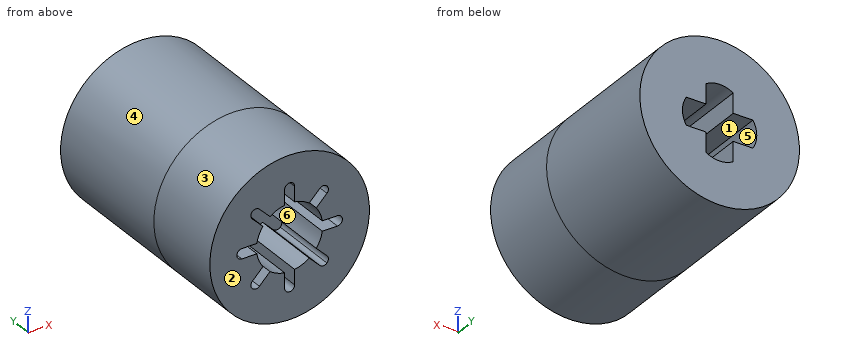
Autodesk Inventor part; units mm, degrees
ref_plane "YZ Plane" through (0, 0, 0) normal (1, 0, 0) x (0, 1, 0)
ref_plane "XZ Plane" through (0, 0, 0) normal (0, 1, 0) x (-1, 0, 0)
ref_plane "XY Plane" through (0, 0, 0) normal (0, 0, 1) x (1, 0, 0)
sketch "Sketch1" plane through (0, 0, 0) normal (0, 1, 0) x (-1, 0, 0)
  arc A0 (0, 3.7886) -> (-0.36, 3.4286) centre (0, 3.4286) ccw
  arc A1 (0.36, 3.4286) -> (0, 3.7886) centre (0, 3.4286) ccw
  line L0 (0, 3.7886) -> (0, 3.7886)
  line L1 (-2.6789, 2.1698) -> (-1.9152, 1.4061)
  arc A2 (-2.1698, 2.6789) -> (-2.6789, 2.6789) centre (-2.4244, 2.4244) ccw
  line L2 (-2.6789, 2.6789) -> (-2.6789, 2.6789)
  arc A3 (-2.6789, 2.6789) -> (-2.6789, 2.1698) centre (-2.4244, 2.4244) ccw
  line L3 (-3.4286, 0.36) -> (-2.3486, 0.36)
  arc A4 (-2.3486, 0.36) -> (-2.3486, -0.36) centre (0, 0) ccw
  line L4 (-3.4286, -0.36) -> (-2.3486, -0.36)
  arc A5 (-3.4286, 0.36) -> (-3.7886, 0) centre (-3.4286, 0) ccw
  line L5 (-3.7886, 0) -> (-3.7886, 0)
  arc A6 (-3.7886, 0) -> (-3.4286, -0.36) centre (-3.4286, 0) ccw
  line L6 (-2.6789, -2.1698) -> (-1.9152, -1.4061)
  arc A7 (-2.6789, -2.1698) -> (-2.6789, -2.6789) centre (-2.4244, -2.4244) ccw
  line L7 (-2.6789, -2.6789) -> (-2.6789, -2.6789)
  arc A8 (-2.6789, -2.6789) -> (-2.1698, -2.6789) centre (-2.4244, -2.4244) ccw
  line L8 (-2.1698, -2.6789) -> (-1.4061, -1.9152)
  arc A9 (-1.9152, -1.4061) -> (-1.4061, -1.9152) centre (0, 0) ccw
  line L9 (-0.36, -3.4286) -> (-0.36, -2.3486)
  arc A10 (-0.36, -2.3486) -> (0.36, -2.3486) centre (0, 0) ccw
  arc A11 (-0.36, -3.4286) -> (0, -3.7886) centre (0, -3.4286) ccw
  line L10 (0, -3.7886) -> (0, -3.7886)
  arc A12 (0, -3.7886) -> (0.36, -3.4286) centre (0, -3.4286) ccw
  line L11 (0.36, -3.4286) -> (0.36, -2.3486)
  line L12 (2.1698, -2.6789) -> (1.4061, -1.9152)
  arc A13 (1.4061, -1.9152) -> (1.9152, -1.4061) centre (0, 0) ccw
  arc A14 (2.1698, -2.6789) -> (2.6789, -2.6789) centre (2.4244, -2.4244) ccw
  line L13 (2.6789, -2.6789) -> (2.6789, -2.6789)
  arc A15 (2.6789, -2.6789) -> (2.6789, -2.1698) centre (2.4244, -2.4244) ccw
  line L14 (2.6789, -2.1698) -> (1.9152, -1.4061)
  line L15 (3.4286, -0.36) -> (2.3486, -0.36)
  arc A16 (2.3486, -0.36) -> (2.3486, 0.36) centre (0, 0) ccw
  line L16 (3.4286, 0.36) -> (2.3486, 0.36)
  arc A17 (3.4286, -0.36) -> (3.7886, 0) centre (3.4286, 0) ccw
  line L17 (3.7886, 0) -> (3.7886, 0)
  arc A18 (3.7886, 0) -> (3.4286, 0.36) centre (3.4286, 0) ccw
  line L18 (2.6789, 2.1698) -> (1.9152, 1.4061)
  arc A19 (1.9152, 1.4061) -> (1.4061, 1.9152) centre (0, 0) ccw
  arc A20 (2.6789, 2.1698) -> (2.6789, 2.6789) centre (2.4244, 2.4244) ccw
  line L19 (2.6789, 2.6789) -> (2.6789, 2.6789)
  arc A21 (2.6789, 2.6789) -> (2.1698, 2.6789) centre (2.4244, 2.4244) ccw
  line L20 (2.1698, 2.6789) -> (1.4061, 1.9152)
  line L21 (0.36, 3.4286) -> (0.36, 2.3486)
  arc A22 (0.36, 2.3486) -> (-0.36, 2.3486) centre (0, 0) ccw
  line L22 (-2.1698, 2.6789) -> (-1.4061, 1.9152)
  arc A23 (-1.4061, 1.9152) -> (-1.9152, 1.4061) centre (0, 0) ccw
  circle A24 centre (0, 0) radius 2.376
  line L23 (-0.36, 3.4286) -> (-0.36, 2.3486)
  circle A25 centre (0, 0) radius 5.7281
  point P0 (-0.36, 3.7886)
  point P1 (0.36, 3.7886)
  point P2 (-2.0323, 2.0323)
  point P3 (-2.9335, 2.4244)
  point P4 (-2.4244, 2.9335)
  point P5 (-3.7886, 0.36)
  point P6 (-2.8742, 0)
  point P7 (-3.7886, -0.36)
  point P8 (-2.9335, -2.4244)
  point P9 (-2.0323, -2.0323)
  point P10 (-2.4244, -2.9335)
  point P11 (-0.36, -3.7886)
  point P12 (0, -2.8742)
  point P13 (0.36, -3.7886)
  point P14 (2.4244, -2.9335)
  point P15 (2.0323, -2.0323)
  point P16 (2.9335, -2.4244)
  point P17 (3.7886, -0.36)
  point P18 (2.8742, 0)
  point P19 (3.7886, 0.36)
  point P20 (2.9335, 2.4244)
  point P21 (2.4244, 2.9335)
  point P22 (2.0323, 2.0323)
  point P23 (0, 2.8742)
  point P24 (-1.4061, 1.9152)
  point P25 (0, 3.7886)
  point P26 (1.4061, 1.9152)
  point P27 (1.9152, 1.4061)
  point P28 (2.3486, 0.36)
  point P29 (3.7886, 0)
  point P30 (2.3486, -0.36)
  point P31 (2.6789, -2.6789)
  point P32 (1.4061, -1.9152)
  point P33 (0.36, -2.3486)
  point P34 (0, -3.7886)
  point P35 (-0.36, -2.3486)
  point P36 (-1.4061, -1.9152)
  point P37 (-2.6789, -2.6789)
  point P38 (-1.9152, -1.4061)
  point P39 (-2.3486, -0.36)
  point P40 (-3.7886, 0)
  point P41 (-1.9152, 1.4061)
  dimension "d2" = 4.752
  dimension "d3" = 0.72
  dimension "d4" = 1.44
  dimension "d5" = 1.44
  dimension "d6" = 0.36
  dimension "d7" = 360
  dimension "d38" = 0
  dimension "d39" = 0
extrude "Extrusion1" add sketch "Sketch1" along normal blind 5
sketch "Sketch2" plane through (0, 5, 0) normal (0, 1, 0) x (1, 0, 0)
  circle A0 centre (0, 0) radius 5.7281
  point P0 (0, 0)
extrude "Extrusion2" add sketch "Sketch2" along normal blind 1
sketch "Sketch7" plane through (0, 6, 0) normal (0, 1, 0) x (1, 0, 0)
  line L0 (2.3926, -0.9756) -> (2.3926, 0.9756)
  line L1 (2.3926, 0.9756) -> (0.9755, 0.9755)
  line L2 (0.9755, 0.9755) -> (0.9754, 2.3926)
  line L3 (0.9754, 2.3926) -> (-0.9756, 2.3926)
  arc A0 (0.9754, 2.3926) -> (-0.9756, 2.3926) centre (0, 0.8054) ccw
  arc A1 (2.3926, -0.9756) -> (2.3926, 0.9756) centre (0.8054, 0) ccw
  line L4 (2.3926, -0.9756) -> (0.9755, -0.9756)
  line L5 (0.9755, -0.9756) -> (0.9756, -2.3926)
  line L6 (0.9756, -2.3926) -> (-0.9755, -2.3926)
  arc A2 (-0.9755, -2.3926) -> (0.9756, -2.3926) centre (0, -0.8054) ccw
  line L7 (-0.9756, 2.3926) -> (-0.9756, 0.9756)
  line L8 (-0.9755, -2.3926) -> (-0.9756, -0.9755)
  line L9 (-0.9756, 0.9756) -> (-2.3926, 0.9756)
  line L10 (-2.3926, 0.9756) -> (-2.3925, -0.9755)
  line L11 (-2.3925, -0.9755) -> (-0.9756, -0.9755)
  arc A3 (-2.3926, 0.9756) -> (-2.3925, -0.9755) centre (-0.8054, 0) ccw
  circle A4 centre (0, 0) radius 5.728
  dimension "d29" = 1.951
  dimension "d32" = 1.9511
  dimension "d34" = 0.9756
  dimension "d31" = 1.4171
  dimension "d30" = 1.417
  dimension "d33" = 2.5838
  dimension "d28" = 1.863
  dimension "d27" = 1.863
  dimension "d25" = 1.417
  dimension "d24" = 1.9511
  dimension "d23" = 1.863
  dimension "d26" = 1.417
  dimension "d21" = 2.5838
  dimension "d20" = 1.9511
  dimension "d19" = 1.863
  dimension "d18" = 2.3925
  dimension "d17" = 2.3925
  dimension "d22" = 1.417
  dimension "d16" = 1.417
  dimension "d15" = 11.456
extrude "Extrusion4" add sketch "Sketch7" along normal blind 10
properties part number "Servo_stycke"
Geometry check sheet. Reference: the model listing, model coordinates, mm. Face numbers are marked on the shaded views. A direction names the side the tool comes from. Give positions to 0.01 mm unless a question says otherwise; leave off trailing zeros. Write each loop counter-clockwise with the first axis right and the second up, starting at its lowest first coordinate (ties: lowest second). Pieces come first, ordered by that corner, then holes. Notation, with made-up numbers: (-24, 19) - (18, 19) arc R14 cw to (18, 38) - close; hole circle Ø9 at (23.5, -33). An arc over 180 degrees is marked (long way). Put each result on its own line as item: value.
1. Draft check along X on the marked faces 1, 2 and 3. Enter one of: +X half, -X half, draft (parallel to the pull), parting line (faces both ways), or undercut.
Ans:
face 1: undercut
face 2: draft
face 3: parting line
2. Thickness scan on line 1 (Z direction, x = 2, y = 7.75); line 2 (Z direction, x = 1.75, y = 14.25); line 3 (X direction, y = 13.5, z = -0.5). Record the ranges inside material, lowest first.
Ans:
line 1: z = -5.37 to -0.98, 0.98 to 5.37
line 2: z = -5.45 to -0.98, 0.98 to 5.45
line 3: x = -5.71 to -2.6, 2.6 to 5.71
3. Sectioned sample at C-C, the plane z = -4.5. Enter the section's corners in (x, y).
Ans:
outline: (-3.54, 0) - (3.54, 0) - (3.54, 16) - (-3.54, 16) - close
4. Set-up check for the marked faces 4, 5 and 6: record each of +Z, -Z, +X, -X, +Y, -Y from which the full face is reachable in a straight line by a thin tool's end or side.
Ans:
face 4: +Y, -Y
face 5: +Y
face 6: -Y
5. Sectioned sample at B-B, the plane z = -3. Enter the section's corners in (x, y).
Ans:
outline: (-4.88, 0) - (-0.36, 0) - (-0.36, 5) - (0.36, 5) - (0.36, 0) - (4.88, 0) - (4.88, 16) - (-4.88, 16) - close
6. Go/stop test with flat-tipped pins: pin 1 (0.5 mm diameter, centred on y = 3, z = -3, fed in from +X); pin 2 (1.1 mm diameter, centred on y = 12.5, z = 1.5, fed in from -X); pin 3 (0.5 mm diameter, centred on x = 3, y = 3, fed in from +Z). Record where each tip stops, or that it passes through.
Ans:
pin 1: stops at x = 5.02
pin 2: stops at x = -5.65
pin 3: stops at z = 5.02
7. Sectioned sample at A-A, the plane y = 8.25. Enter the section's corners in (x, z), plus the area to 3 significant figures.
Ans:
outline: circle Ø11.46 at (0, 0); hole (-2.39, -0.98) - (-0.98, -0.98) - (-0.98, -2.39) arc R1.86 ccw to (0.98, -2.39) - (0.98, -0.98) - (2.39, -0.98) arc R1.86 ccw to (2.39, 0.98) - (0.98, 0.98) - (0.98, 2.39) arc R1.86 ccw to (-0.98, 2.39) - (-0.98, 0.98) - (-2.39, 0.98) arc R1.86 ccw to start
area: 86.8 mm²
